Input: part model. Units: mm. Frame: model coordinates. A direction names the side the tool comes from. Round coordinates to 2 decimals unless told otherwise and drop trailing zeros. Loops run counter-clockwise (first coordinate to the right, second up) from the corner with the lowest first, then second, coordinate; pieces in that order, holes last.
1) Section C-C, the plane x = -4. Return loops of the section in (y, z).
2) Section A-A, the plane z = 169.5. Return loops of the section in (x, y).
3) Ray query, line 1 along Y through (x, z) = (-7, 99); line 2 along X through (y, z) = (-5.25, 48). Return the intervals inside material, ascending.
4) Draft query along X for faces 1 (the face through (12, 0, 100)), 2 (the face through (13.289, -13.196, 103.803)), 3 (the face through (-15, 0, 166)), 4 (the face through (0, 15, 130)). Return one class per face: pulls with the +X half, pulls with the -X half, needs draft (parallel to the pull), parting line crosses it, or undercut.
5) Access query for faces 5 (the face through (0, 12, 130)), 6 (the face through (-13.196, -13.289, 157.84)). Directions: +Z, -Z, +X, -X, +Y, -Y. A direction counts if a zero-diameter tool reaches every point of the face in a straight line with its end or side. Return the directions, or none.
6) Section B-B, the plane y = 1. Return loops of the section in (x, z), and give its area (3 significant figures).
7) Section D-D, the plane z = 227. Return loops of the section in (x, y).
Autodesk Inventor part; units mm, degrees
ref_plane "Start Plane" through (0, 0, 19.0291) normal (0, 0, 1) x (1, 0, 0)
ref_plane "End Plane" through (0, 0, 245.024) normal (0, 0, 1) x (1, 0, 0)
ref_plane "Work Plane4" through (52.8262, -9, -108.7856) normal (-0.9468, 0, -0.3219) x (-0.3219, 0, 0.9468)
ref_plane "Start Plane" through (0, 0, 19.0291) normal (0, 0, 1) x (1, 0, 0)
ref_plane "End Plane" through (0, 0, 245.024) normal (0, 0, 1) x (1, 0, 0)
sketch "Sketch" plane through (0, 0, 0) normal (0, 0, 1) x (1, 0, 0)
  line L0 (-15, -9) -> (-15, 9)
  line L1 (-9, 15) -> (9, 15)
  line L2 (15, 9) -> (15, -9)
  line L3 (9, -15) -> (-9, -15)
  arc A0 (-15, -9) -> (-9, -15) centre (-9, -9) ccw
  arc A1 (-9, 15) -> (-15, 9) centre (-9, 9) ccw
  arc A2 (15, 9) -> (9, 15) centre (9, 9) ccw
  arc A3 (9, -15) -> (15, -9) centre (9, -9) ccw
  arc A4 (-9, 12) -> (-12, 9) centre (-9, 9) ccw
  line L4 (-9, 12) -> (9, 12)
  arc A5 (12, 9) -> (9, 12) centre (9, 9) ccw
  line L5 (12, 9) -> (12, -9)
  arc A6 (9, -12) -> (12, -9) centre (9, -9) ccw
  line L6 (9, -12) -> (-9, -12)
  arc A7 (-12, -9) -> (-9, -12) centre (-9, -9) ccw
  line L7 (-12, -9) -> (-12, 9)
  line L8 (0, 22.7397) -> (0, -22.7397) construction
  line L9 (-22.7397, 0) -> (22.7397, 0) construction
  dimension "d7" = 6
  dimension "d10" = 30
  dimension "d11" = 30
  dimension "d12" = 3
  dimension "d15" = 15
  dimension "d16" = 15
extrude "Body" add sketch "Sketch" along normal up to surface (225.9948 mm away) from surface at 19.0291
sketch "Sketch3" plane through (0, 0, 0) normal (0, 0, 1) x (1, 0, 0)
  line L0 (0, 0) -> (10, 0)
ref_plane "Work Plane3" through (0, 0, 0) normal (0, -1, 0) x (1, 0, 0)
ref_plane "Work Plane4" through (52.8262, -9, -108.7856) normal (-0.9468, 0, -0.3219) x (-0.3219, 0, 0.9468)
split "Split1" plane through (52.8262, -9, -108.7856) removes the side toward (-0.9468, 0, -0.3219)
ref_plane "Work Plane5" through (75.6449, 9, 41.5617) normal (0.3219, 0, -0.9468) x (-0.9468, 0, -0.3219)
split "Split2" plane through (75.6449, 9, 41.5617) removes the side toward (0.3219, 0, -0.9468)
ref_plane "Work Plane6" through (-14.2016, 9, 259.2256) normal (0.9468, 0, 0.3219) x (0.3219, 0, -0.9468)
split "Split3" plane through (-14.2016, 9, 259.2256) removes the side toward (0.9468, 0, 0.3219)
ref_plane "Work Plane7" through (4.8284, -9, 249.8524) normal (-0.3219, 0, 0.9468) x (0.9468, 0, 0.3219)
split "Split4" plane through (4.8284, -9, 249.8524) removes the side toward (-0.3219, 0, 0.9468)
sketch "Sketch4" plane through (0, 0, 0) normal (0, -1, 0) x (1, 0, 0)
  line L0 (-2, 19.0291) -> (12, 19.0291)
  line L1 (-2, 245.024) -> (12, 245.024)
  dimension "d18" = 225.9948
equation "\"d7\" = G_IR"
equation "\"d10\" = G_H"
equation "\"d11\" = G_W"
equation "\"d12\" = G_T"
equation "\"d15\" = 0.5 * d10"
equation "\"d16\" = 0.5 * d11"
equation "\"d3\" = G_L"
equation "\"G_W\" = 30"
equation "\"G_H\" = 30"
equation "\"G_T\" = 3"
equation "\"G_IR\" = 6"
equation "\"G_L\" = d18"
equation "\"G_OFFSET_START\" = -19.02914"
equation "\"G_OFFSET_END\" = -19.03004"
equation "\"d13\" = -G_OFFSET_START"
equation "\"d14\" = G_OFFSET_END + B_L"
equation "\"B_L\" = 264.05402"
properties part number "DIN EN 10219-2 - 30 x 30 x 3  - 225.99" material "Steel, Mild"
Final values:
1. outline: (-15, 58.36) - (-12, 58.36) - (-12, 229.22) - (-15, 229.22) - close; (12, 58.36) - (15, 58.36) - (15, 229.22) - (12, 229.22) - close
2. outline: (-15, -9) arc R6 ccw to (-9, -15) - (9, -15) arc R6 ccw to (15, -9) - (15, 9) arc R6 ccw to (9, 15) - (-9, 15) arc R6 ccw to (-15, 9) - close; hole (-12, -9) arc R3 ccw to (-9, -12) - (9, -12) arc R3 ccw to (12, -9) - (12, 9) arc R3 ccw to (9, 12) - (-9, 12) arc R3 ccw to (-12, 9) - close
3. line 1: y = -15 to -12, 12 to 15
3. line 2: x = 12 to 15
4. face 1: undercut
4. face 2: pulls with the +X half
4. face 3: pulls with the -X half
4. face 4: needs draft
5. face 5: +Z, -Z
5. face 6: +Z, -Z, -X, -Y
6. outline: (-15, 90.71) - (-12, 81.89) - (-12, 244.13) - (-15, 243.11) - close; (12, 19.92) - (15, 20.94) - (15, 173.34) - (12, 182.16) - close
6. area: 944 mm2
7. outline: (-15, -9) arc R6 ccw to (-9, -15) - (-3.25, -15) - (-3.25, -12) - (-9, -12) arc R3 cw to (-12, -9) - (-12, 9) arc R3 cw to (-9, 12) - (-3.25, 12) - (-3.25, 15) - (-9, 15) arc R6 ccw to (-15, 9) - close
